The listing builds one solid part. Answer for the finished solid, in the listing's coordinates (mm). Face numbers are marked on the shaded views. A direction names the side the tool comes from. Round coordinates to 2 decimals unless told otherwise and drop trailing zeros. Loops run counter-clockwise (first coordinate to the right, second up) from the corner with the lowest first, then second, coordinate; pieces in that order, holes last. Notation, with made-up numbers: (58, -33.75) -> (113, -33.75) arc R33 cw to (113, 0.25) -> close; hole circle Ø5 at (30, 57.5). An arc over 180 degrees is marked (long way). Use a Markdown table: item, result. Add a question column.
Q1. Section D-D on z = 16 is taken. Give the vertices of the cut face in (x, y).
Q2. Section C-C on x = 10.5 is taken. Give the vertices of the cut face in (y, z), then the cut area to 3 significant figures.
Q3. Which of the six approach directions +Z, -Z, +X, -X, +Y, -Y give full straight-line access (tool end or side, diameter ignored) to the marked faces 1 and 2?
Q4. Section B-B on z = 25 is taken. Give the vertices of the cut face in (x, y), then the cut area to 3 significant figures.
Q5. Given pin 1 Ø1 at (y, z) = (5.5, -18.5) entering from +X; pin 2 Ø8 at (x, z) = (7.5, -24) entering from +Y; pin 3 Ø9 at (x, z) = (10.5, -25) entering from +Y, each flat-ended and moving along its own axis, determine where each tip first touches the part or whether it passes through.
Q6. Consider line 1 (Y direction, x = 8, z = 2.5); line 2 (X direction, y = 1.65, z = 25). Determine where each line is inside the solid, lowest interval first.
Q7. Section A-A on y = 8 is taken. Give the vertices of the cut face in (x, z).
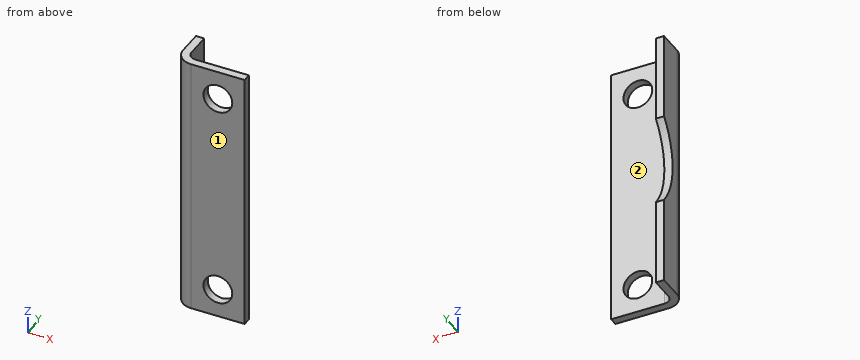
from build123d import *

# Parameters (mm, degrees)
EXTRUDE_1_DEPTH     = 32
FILLET_1_R          = 4
FILLET_2_R          = 2
SKETCH_2_R          = 3.5
CUT_EXTRUDE_1_DEPTH = 10
SKETCH_3_R          = 17
CUT_EXTRUDE_2_DEPTH = 10


with BuildPart() as part:
    # 草图1 → 凸台-拉伸1 (new, symmetric)
    with BuildSketch(Plane.XY):
        Polygon((0, 0), (0, 10), (2, 10), (2, 2), (17, 2), (17, 0), align=None)
    extrude(amount=EXTRUDE_1_DEPTH, both=True)

    # 圆角1
    fillet_1_edges = [part.edges().sort_by_distance(p)[0] for p in [
        (0, 0, 0),
    ]]
    fillet(fillet_1_edges, radius=FILLET_1_R)

    # 圆角2
    fillet_2_edges = [part.edges().sort_by_distance(p)[0] for p in [
        (2, 2, 0),
    ]]
    fillet(fillet_2_edges, radius=FILLET_2_R)

    # 草图2 → 切除-拉伸1 (cut)
    with BuildSketch(Plane.XZ):
        with Locations(Location((10.5, 25, 0), (0, 0, 270))):
            Circle(SKETCH_2_R)
        with Locations((10.5, -25)):
            Circle(SKETCH_2_R)
    extrude(amount=-CUT_EXTRUDE_1_DEPTH, mode=Mode.SUBTRACT)

    # 草图3 → 切除-拉伸2 (cut)
    with BuildSketch(Plane.ZY):
        with Locations((0, 23)):
            Circle(SKETCH_3_R)
    extrude(amount=-CUT_EXTRUDE_2_DEPTH, mode=Mode.SUBTRACT)


solid = part.part
Checked values:
| question | item | result |
|---|---|---|
| 1 | outline | (0, 4) arc R4 ccw to (4, 0) -> (17, 0) -> (17, 2) -> (4, 2) arc R2 cw to (2, 4) -> (2, 10) -> (0, 10) -> close |
| 2 | outline | (0, -32) -> (2, -32) -> (2, -28.5) -> (0, -28.5) -> close; (0, -21.5) -> (2, -21.5) -> (2, 21.5) -> (0, 21.5) -> close; (0, 28.5) -> (2, 28.5) -> (2, 32) -> (0, 32) -> close |
| 2 | area | 100 mm2 |
| 3 | face 1 | +Z, -Z, +X, -X, -Y |
| 3 | face 2 | +Z, -Z, +X, +Y |
| 4 | outline | (0, 4) arc R4 ccw to (4, 0) -> (7, 0) -> (7, 2) -> (4, 2) arc R2 cw to (2, 4) -> (2, 10) -> (0, 10) -> close; (14, 0) -> (17, 0) -> (17, 2) -> (14, 2) -> close |
| 4 | area | 33.4 mm2 |
| 5 | pin 1 | stops at x = 2 |
| 5 | pin 2 | stops at y = 2.06 |
| 5 | pin 3 | stops at y = 2 |
| 6 | line 1 | y = 0 to 2 |
| 6 | line 2 | x = 0.76 to 7, 14 to 17 |
| 7 | outline | (0, -32) -> (2, -32) -> (2, -8) -> (0, -8) -> close; (0, 8) -> (2, 8) -> (2, 32) -> (0, 32) -> close |
